Design review of the part built by this model. Coordinates are the model's own, in mm. A direction names the side the tool comes from. Coordinates: 2 decimals unless noted, no trailing zeros. Loops run counter-clockwise (first coordinate to the right, second up) from the corner with the lowest first, then second, coordinate; pieces in that order, holes last. Notation, with made-up numbers: (3, 9) -> (44, 9) arc R35 ccw to (44, 45) -> close; hole circle Ø6 at (63, 79.5). An arc over 180 degrees is marked (long way). Answer as a JSON object with one key per item and string values.
```python
from build123d import *

# Parameters (mm, degrees)
SKETCH3_R               = 2.1
SALIENTE_EXTRUIR1_DEPTH = 200


with BuildPart() as part:
    # Sketch3 → Saliente-Extruir1 (new body)
    with BuildSketch(Plane(origin=(0, 0, 0), x_dir=(1, 0, 0), z_dir=(0, 1, 0))):
        with BuildLine():
            Line((-19.2, -10), (-14.728647189, -10))
            Line((-14.728647189, -10), (-12.928647189, -8.2))
            Line((-12.928647189, -8.2), (-15.179339828, -8.2))
            Line((-15.179339828, -8.2), (-15.179339828, -6.24))
            Line((-15.179339828, -6.24), (-12.84, -3.900660172))
            Line((-12.84, -3.900660172), (-7.16, -3.900660172))
            Line((-7.16, -3.900660172), (-4.820660172, -6.24))
            Line((-4.820660172, -6.24), (-4.820660172, -8.2))
            Line((-4.820660172, -8.2), (-7.104380066, -8.2))
            Line((-7.104380066, -8.2), (-5.304380066, -10))
            Line((-5.304380066, -10), (0, -10))
            Line((0, -10), (5.304380066, -10))
            Line((5.304380066, -10), (7.104380066, -8.2))
            Line((7.104380066, -8.2), (4.820660172, -8.2))
            Line((4.820660172, -8.2), (4.820660172, -6.24))
            Line((4.820660172, -6.24), (7.16, -3.900660172))
            Line((7.16, -3.900660172), (12.84, -3.900660172))
            Line((12.84, -3.900660172), (15.179339828, -6.24))
            Line((15.179339828, -6.24), (15.179339828, -8.2))
            Line((15.179339828, -8.2), (12.928647189, -8.2))
            Line((12.928647189, -8.2), (14.728647189, -10))
            Line((14.728647189, -10), (19.2, -10))
            ThreePointArc((19.2, -10), (19.765685425, -9.765685425), (20, -9.2))
            Line((20, -9.2), (20, -4.619288759))
            Line((20, -4.619288759), (18.2, -2.819288759))
            Line((18.2, -2.819288759), (18.2, -5.179339828))
            Line((18.2, -5.179339828), (16.24, -5.179339828))
            Line((16.24, -5.179339828), (13.900660172, -2.84))
            Line((13.900660172, -2.84), (13.900660172, 2.84))
            Line((13.900660172, 2.84), (16.24, 5.179339828))
            Line((16.24, 5.179339828), (18.2, 5.179339828))
            Line((18.2, 5.179339828), (18.2, 2.895619934))
            Line((18.2, 2.895619934), (20, 4.695619934))
            Line((20, 4.695619934), (20, 9.2))
            ThreePointArc((20, 9.2), (19.765685425, 9.765685425), (19.2, 10))
            Line((19.2, 10), (14.652316014, 10))
            Line((14.652316014, 10), (12.852316014, 8.2))
            Line((12.852316014, 8.2), (15.179339828, 8.2))
            Line((15.179339828, 8.2), (15.179339828, 6.24))
            Line((15.179339828, 6.24), (12.84, 3.900660172))
            Line((12.84, 3.900660172), (7.16, 3.900660172))
            Line((7.16, 3.900660172), (4.820660172, 6.24))
            Line((4.820660172, 6.24), (4.820660172, 8.2))
            Line((4.820660172, 8.2), (7.180711241, 8.2))
            Line((7.180711241, 8.2), (5.380711241, 10))
            Line((5.380711241, 10), (0, 10))
            Line((0, 10), (-5.380711241, 10))
            Line((-5.380711241, 10), (-7.180711241, 8.2))
            Line((-7.180711241, 8.2), (-4.820660172, 8.2))
            Line((-4.820660172, 8.2), (-4.820660172, 6.24))
            Line((-4.820660172, 6.24), (-7.16, 3.900660172))
            Line((-7.16, 3.900660172), (-12.84, 3.900660172))
            Line((-12.84, 3.900660172), (-15.179339828, 6.24))
            Line((-15.179339828, 6.24), (-15.179339828, 8.2))
            Line((-15.179339828, 8.2), (-12.852316014, 8.2))
            Line((-12.852316014, 8.2), (-14.652316014, 10))
            Line((-14.652316014, 10), (-19.2, 10))
            ThreePointArc((-19.2, 10), (-19.765685425, 9.765685425), (-20, 9.2))
            Line((-20, 9.2), (-20, 4.695619934))
            Line((-20, 4.695619934), (-18.2, 2.895619934))
            Line((-18.2, 2.895619934), (-18.2, 5.179339828))
            Line((-18.2, 5.179339828), (-16.24, 5.179339828))
            Line((-16.24, 5.179339828), (-13.900660172, 2.84))
            Line((-13.900660172, 2.84), (-13.900660172, -2.84))
            Line((-13.900660172, -2.84), (-16.24, -5.179339828))
            Line((-16.24, -5.179339828), (-18.2, -5.179339828))
            Line((-18.2, -5.179339828), (-18.2, -2.819288759))
            Line((-18.2, -2.819288759), (-20, -4.619288759))
            Line((-20, -4.619288759), (-20, -9.2))
            ThreePointArc((-20, -9.2), (-19.765685425, -9.765685425), (-19.2, -10))
        make_face()
        with Locations(Location((-10, 0, 0), (0, 0, 270))):
            Circle(SKETCH3_R, mode=Mode.SUBTRACT)
        with Locations(Location((10, 0, 0), (0, 0, 270))):
            Circle(SKETCH3_R, mode=Mode.SUBTRACT)
        Polygon((-2.699339828, -6.24), (-6.099339828, -2.84), (-6.099339828, 2.84), (-2.699339828, 6.24), (-2.699339828, 8.2), (2.699339828, 8.2), (2.699339828, 6.24), (6.099339828, 2.84), (6.099339828, -2.84), (2.699339828, -6.24), (2.699339828, -8.2), (-2.699339828, -8.2), align=None, mode=Mode.SUBTRACT)
    extrude(amount=SALIENTE_EXTRUIR1_DEPTH)


solid = part.part
```
1) The part is to be moulded in two halves that separate along Z. For faces 1 (the flat face through (4.38, 98.6, -4.56)), 2 (the flat face through (-10, 99, 3.901)), 3 (the flat face through (-10, 99, -3.901)), say which applies: pulls with the +Z half, pulls with the -Z half, needs draft (parallel to the pull), parting line crosses it, or undercut.
Completed:
{"face 1": "undercut", "face 2": "pulls with the +Z half", "face 3": "pulls with the -Z half"}
2) Add section B-B, the plane x = -10. Give the boundary of the cut face in (y, z).
Completed:
{"outline": "(0, -3.9) -> (200, -3.9) -> (200, -2.1) -> (0, -2.1) -> close; (0, 2.1) -> (200, 2.1) -> (200, 3.9) -> (0, 3.9) -> close"}
3) Add section A-A, the plane z = 0. Give the boundary of the cut face in (x, y), and give its area (3 significant figures).
Completed:
{"outline": "(-13.9, 0) -> (-12.1, 0) -> (-12.1, 200) -> (-13.9, 200) -> close; (-7.9, 0) -> (-6.1, 0) -> (-6.1, 200) -> (-7.9, 200) -> close; (6.1, 0) -> (7.9, 0) -> (7.9, 200) -> (6.1, 200) -> close; (12.1, 0) -> (13.9, 0) -> (13.9, 200) -> (12.1, 200) -> close", "area": "1,440 mm²"}
4) Add section C-C, the plane y = 48. Count the separate pieces of the cut face and the enclosed holes in it, and give its area (3 significant figures).
Completed:
{"separate pieces": "1", "enclosed holes": "3", "area": "306 mm²"}
5) Clearance check with flat-ended pins moving along their axes: pin 1 Ø1.7 at (y, z) = (54, 0.5) entering from +X; pin 2 Ø1.7 at (x, y) = (10.5, 114) entering from +Z; pin 3 Ø6 at (x, y) = (10.5, 145) entering from -Z. State where each tip first meets the part, or that it passes through.
Completed:
{"pin 1": "x = 13.9", "pin 2": "z = 3.9", "pin 3": "z = -8.85"}
6) Wall thickness on probe 1 along X at (y, z) = (105, 0); probe 2 along Z at (x, y) = (5, 157.5); probe 3 along X at (y, z) = (139.5, -6.5): over which ranges is each line inside the solid? List them lowest first.
Completed:
{"probe 1": "-13.9 to -12.1, -7.9 to -6.1, 6.1 to 7.9, 12.1 to 13.9", "probe 2": "-10 to -8.2, -6.06 to -3.94, 3.94 to 6.06, 8.2 to 10", "probe 3": "-20 to -15.18, -4.82 to -2.7, 2.7 to 4.82, 15.18 to 20"}
7) For faces 4 (the flat face through (-13.901, 99, 0)), 5 (the flat face through (0, 99, -8.2)), 6 (the flat face through (10, 99, 3.901)), 7 (the flat face through (-5, 0, -5)), 8 (the flat face through (10, 99, -3.901)), list the 3-axis set-ups (+Z, -Z, +X, -X, +Y, -Y) from which the entire face can be reached by the end or side of a thin tool; tool diameter is ignored.
Completed:
{"face 4": "-X, +Y, -Y", "face 5": "+Y, -Y", "face 6": "+Z, +Y, -Y", "face 7": "+Z, -Z, +X, -X, -Y", "face 8": "-Z, +Y, -Y"}
